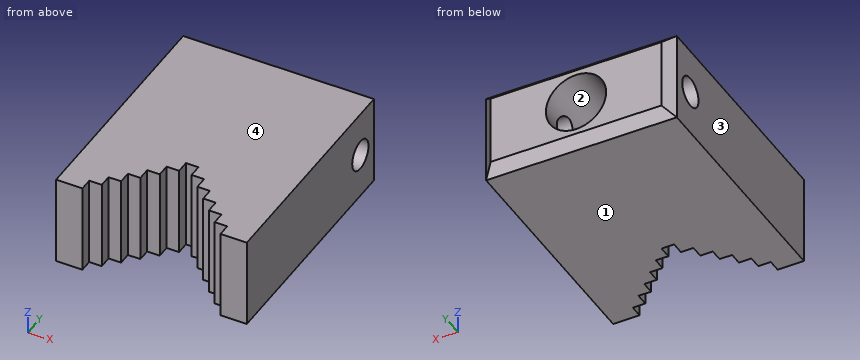
```python
from build123d import *

# Parameters (mm, degrees)
BOSS_EXTRUDE1_DEPTH       = 18
CHAMFER1_SIZE             = 2
CUT_EXTRUDE1_DEPTH        = 49.624263051
CUT_EXTRUDE1_DEPTH_BACK   = 49.624263051
SKETCH3_R                 = 3
F_1_0MM_DOWEL_HOLE1_D     = 12
F_1_0MM_DOWEL_HOLE1_DEPTH = 20
F_1_0MM_DOWEL_HOLE1_TIP   = 3.464101615


with BuildPart() as part:
    # Sketch1 → Boss-Extrude1 (new body)
    with BuildSketch(Plane.XY):
        Polygon((-13.75, -24.419642857), (-13.75, -21.919642857), (-11.25, -21.919642857), (-11.25, -19.419642857), (-8.75, -19.419642857), (-8.75, -16.919642857), (-6.25, -16.919642857), (-6.25, -14.419642857), (-3.75, -14.419642857), (-3.75, -11.919642857), (-1.25, -11.919642857), (-1.25, -9.419642857), (1.25, -9.419642857), (1.25, -11.919642857), (3.75, -11.919642857), (3.75, -14.419642857), (6.25, -14.419642857), (6.25, -16.919642857), (8.75, -16.919642857), (8.75, -19.419642857), (11.25, -19.419642857), (11.25, -21.919642857), (13.75, -21.919642857), (13.75, -24.419642857), (19, -24.419642857), (19, 24.419642857), (-19, 24.419642857), (-19, -24.419642857), align=None)
    extrude(amount=BOSS_EXTRUDE1_DEPTH)

    # Chamfer1
    chamfer1_edges = [part.edges().sort_by_distance(p)[0] for p in [
        (0, 24.419642857, 0),
        (-19, 24.419642857, 9),
        (19, 24.419642857, 9),
        (0, 24.419642857, 18),
    ]]
    chamfer(chamfer1_edges, length=CHAMFER1_SIZE)

    # Sketch3 → Cut-Extrude1 (cut, two sides: drawn at the far end of the back side and taken through both)
    with BuildSketch(Plane(origin=(19, 0, 0), x_dir=(0, 0, -1), z_dir=(1, 0, 0)).offset(-CUT_EXTRUDE1_DEPTH_BACK)):
        with Locations((-9, 17.419642857)):
            Circle(SKETCH3_R)
    extrude(amount=CUT_EXTRUDE1_DEPTH + CUT_EXTRUDE1_DEPTH_BACK, mode=Mode.SUBTRACT)

    # Ø1.0mm Dowel Hole1
    with Locations(Plane(origin=(0, 24.419642857, 0), x_dir=(1, 0, 0), z_dir=(0, 1, 0))):
        with Locations((0, -9)):
            Hole(F_1_0MM_DOWEL_HOLE1_D / 2, depth=F_1_0MM_DOWEL_HOLE1_DEPTH)
            with Locations((0, 0, -(F_1_0MM_DOWEL_HOLE1_DEPTH + F_1_0MM_DOWEL_HOLE1_TIP / 2))):  # 120° drill point
                Cone(0, F_1_0MM_DOWEL_HOLE1_D / 2, F_1_0MM_DOWEL_HOLE1_TIP, mode=Mode.SUBTRACT)


solid = part.part
```
Design review of the part built by this model. Coordinates are the model's own, in mm. Face numbers are marked on the shaded views. Coordinates: 2 decimals unless noted, no trailing zeros. Order: outer loops, then holes, each group sorted by start corner. A loop starts at its lowest first (then second) coordinate and runs counter-clockwise, first axis right, second up.
1) Wall thickness on line 1 along X through (y, z) = (-22, 3.75); line 2 along Y through (x, z) = (13, 9); line 3 along Z through (x, y) = (0, 20.75): over which ranges is each line inside the solid? List them lowest first.
2) Clearance check with flat-ended pins moving along their axes: pin 1 (0.8 mm diameter, centred on x = -10.5, z = 8, fed in from -Y); pin 2 (2 mm diameter, centred on x = 7.5, z = 6, fed in from -Y); pin 3 (1.2 mm diameter, centred on x = -12.5, z = 10.5, fed in from -Y). State where each tip first meets the part, or that it passes through.
3) Take a section at A-A, the plane y = -21. Give the boundary of the cut face in (x, z).
4) Take a section at B-B, the plane y = 7. Give the boundary of the cut face in (x, z).
5) Mouldability with a two-part tool opening along Z and no side actions: class the marked faces 1, 2, 3 and 4 as +Z half, -Z half, draft (parallel to the pull), parting line (faces both ways), or undercut.
6) Take a section at C-C, the plane x = 12.5. Give the boundary of the cut face in (y, z).
Returned:
1. line 1: x = -19 to -13.75, 13.75 to 19
1. line 2: y = -21.92 to 14.42, 20.42 to 24.42
1. line 3: z = 0 to 3, 15 to 18
2. pin 1: stops at y = -19.42
2. pin 2: stops at y = -16.92
2. pin 3: stops at y = -21.92
3. outline: (-19, 0) - (-11.25, 0) - (-11.25, 18) - (-19, 18) - close; (11.25, 0) - (19, 0) - (19, 18) - (11.25, 18) - close
4. outline: (-19, 0) - (19, 0) - (19, 18) - (-19, 18) - close; hole circle Ø12 at (0, 9)
5. face 1: -Z half
5. face 2: undercut
5. face 3: draft
5. face 4: +Z half
6. outline: (-21.92, 0) - (22.42, 0) - (24.42, 2) - (24.42, 16) - (22.42, 18) - (-21.92, 18) - close; hole circle Ø6 at (17.42, 9)
